Read the model definition and answer for the solid it produces. Units are mm, in the model's axes. A direction names the side the tool comes from. Give positions to 0.01 mm unless a question says otherwise; leave off trailing zeros. Write each loop counter-clockwise with the first axis right and the second up, starting at its lowest first coordinate (ties: lowest second). Pieces come first, ordered by that corner, then holes. Notation, with made-up numbers: M -29,87.25 L 23,87.25 A33 cw 23,117.25 Z; hole C 1,-12.5 d5. An arc over 180 degrees is marked long. Put each result on its own line as item: value.
Autodesk Inventor part; units mm, degrees
ref_plane "YZ Plane" through (0, 0, 0) normal (1, 0, 0) x (0, 1, 0)
ref_plane "XZ Plane" through (0, 0, 0) normal (0, 1, 0) x (-1, 0, 0)
ref_plane "XY Plane" through (0, 0, 0) normal (0, 0, 1) x (1, 0, 0)
sketch "Sketch1" plane through (0, 0, 0) normal (0, 1, 0) x (-1, 0, 0)
  line L0 (25.4, -10) -> (-25.4, -10)
  line L1 (-25.4, -10) -> (-25.4, 10)
  line L2 (-25.4, 10) -> (25.4, 10)
  line L3 (25.4, 10) -> (25.4, -10)
  line L4 (25.4, -10) -> (-25.4, 10) construction
  line L5 (-25.4, -10) -> (25.4, 10) construction
  circle A0 centre (-17.9, 0) radius 2.5
  circle A1 centre (17.9, 0) radius 2.5
  point P0 (0, 0)
  dimension "d0" = 50.8
  dimension "d1" = 20
  dimension "d2" = 5
  dimension "d3" = 5
  dimension "d4" = 7.5
  dimension "d5" = 7.5
extrude "Extrusion1" add sketch "Sketch1" along normal blind 5.08
ref_plane "Work Plane1" through (0, 0, -10) normal (-1, 0, 0) x (0, 0, 1)
sketch "Sketch2" plane through (0, 0, -10) normal (-1, 0, 0) x (0, 0, 1)
  line L0 (0, 0) -> (20, 0)
  line L1 (0, 0) -> (0, 5.08)
  line L2 (20, 5.08) -> (0, 5.08)
  line L3 (20, 0) -> (20, 5.08)
  line L4 (0, 5.08) -> (20, 5.08)
  line L5 (10, 0) -> (10, 2.54)
  line L6 (10, 5.08) -> (10, 11.43)
  line L7 (10, 11.43) -> (10, 18.93)
  circle A0 centre (10, 18.93) radius 7.5
  line L8 (20, 5.08) -> (20, 18.93)
  line L9 (0, 5.08) -> (0, 18.93)
  arc A1 (20, 18.93) -> (0, 18.93) centre (10, 18.93) ccw
  line L10 (20, 18.93) -> (20, 5.08)
  line L11 (20, 5.08) -> (0, 5.08)
  line L12 (0, 5.08) -> (0, 18.93)
  dimension "d10" = 2.54
  dimension "d11" = 6.35
  dimension "d12" = 7.5
  dimension "d13" = 15
extrude "Extrusion2" add sketch "Sketch2" along normal mid plane 24 contours L9 A1 L8 L2
sketch "Sketch3" plane through (12, 0, -10) normal (1, 0, 0) x (0, 0, -1)
  circle A0 centre (-10, 18.93) radius 7.5
  line L0 (0, 5.08) -> (-20, 5.08)
  line L1 (0, 5.08) -> (0, 18.93)
  arc A1 (0, 18.93) -> (-20, 18.93) centre (-10, 18.93) ccw
  line L2 (-20, 18.93) -> (-20, 5.08)
  circle A2 centre (-10, 18.93) radius 5
  point P0 (-10, 0)
  dimension "d16" = 10
extrude "Extrusion3" add sketch "Sketch3" along normal blind 1 contours A0 | L0 L2 A1 L1
sketch "Sketch4" plane through (-12, 0, -10) normal (-1, 0, 0) x (0, 0, 1)
  circle A0 centre (10, 18.93) radius 7.5
  line L0 (20, 5.08) -> (0, 5.08)
  line L1 (20, 5.08) -> (20, 18.93)
  arc A1 (20, 18.93) -> (0, 18.93) centre (10, 18.93) ccw
  line L2 (0, 18.93) -> (0, 5.08)
  point P0 (10, 0)
extrude "Extrusion4" add sketch "Sketch4" along normal blind 1
(1) Section C-C on y = 15.5 is taken. Determine the outline of the cut face in (x, z), and give its area (3 significant figures).
Result:
outline: M -13,-10 L 13,-10 L 13,-3.64 L 12,-3.64 L 12,-6.67 L -13,-6.67 Z; M -13,6.67 L 12,6.67 L 12,3.64 L 13,3.64 L 13,10 L -13,10 Z
area: 179 mm²
(2) Section B-B on z = 0 is taken. Determine the outline of the cut face in (x, y).
Result:
outline: M -25.4,0 L -20.4,0 L -20.4,5.08 L -25.4,5.08 Z; M -15.4,0 L 15.4,0 L 15.4,5.08 L 13,5.08 L 13,13.93 L 12,13.93 L 12,11.43 L -13,11.43 L -13,5.08 L -15.4,5.08 Z; M -13,26.43 L 12,26.43 L 12,23.93 L 13,23.93 L 13,28.93 L -13,28.93 Z; M 20.4,0 L 25.4,0 L 25.4,5.08 L 20.4,5.08 Z
(3) For a pull along Y with two mould halves and no side action, classify faces 6 (the face through (-20.21, 2.5, 0.96)), 7 (the face through (0, 0, 0)), 8 (the face through (12, 17, -5)), 9 (the face through (-19.1, 5.08, 2.4)) as +Y half, -Y half, draft (parallel to the pull), parting line (faces both ways), or undercut.
Result:
face 6: draft
face 7: -Y half
face 8: undercut
face 9: +Y half
(4) Section D-D on x = 10 is taken. Determine the outline of the cut face in (y, z).
Result:
outline: M 0,-10 L 18.93,-10 A10 ccw 18.93,10 L 0,10 Z; hole C 18.93,0 d15
(5) Section A-A on x = -17.9 is taken. Determine the outline of the cut face in (y, z).
Result:
outline: M 0,-10 L 5.08,-10 L 5.08,-2.5 L 0,-2.5 Z; M 0,2.5 L 5.08,2.5 L 5.08,10 L 0,10 Z
(6) Given pin 1 Ø8 at (x, y) = (-13, 26) entering from +Z; pin 2 Ø4 at (x, z) = (-8, -2.5) entering from -Y; pin 3 Ø4 at (x, z) = (-13, 3) entering from +Y; pin 4 Ø6 at (y, z) = (12.5, 3.5) entering from +X, each flat-ended and moving along its own axis, determine where each tip first touches the part or whether it passes through.
Result:
pin 1: stops at z = 9.52
pin 2: stops at y = 0
pin 3: stops at y = 28.88
pin 4: stops at x = 13
(7) Which of the six approach directions +Z, -Z, +X, -X, +Y, -Y give full straight-line access (tool end or side, diameter ignored) to faces 1 (the face through (13, 12, 0)), 2 (the face through (-13, 12, -5)), 3 (the face through (19.74, 2.5, -1.69)), 4 (the face through (-25.4, 3, 0)), 5 (the face through (-0.32, 26.25, -1.63))?
Result:
face 1: +Z, -Z, +X, +Y
face 2: +Z, -Z, -X, +Y
face 3: +Y, -Y
face 4: +Z, -Z, -X, +Y, -Y
face 5: -X
(8) Straight lines are drawn through the part: line 1 along Z through (x, y) = (-17.9, 2.35); line 2 along Y through (x, z) = (2.5, 0); line 3 along Z through (x, y) = (-3.5, 18.93). For each, find the intervals that lie inside material, in ascending order. Write a range as from..to.
Result:
line 1: z = -10..-2.5, 2.5..10
line 2: y = 0..11.43, 26.43..28.93
line 3: z = -10..-7.5, 7.5..10
